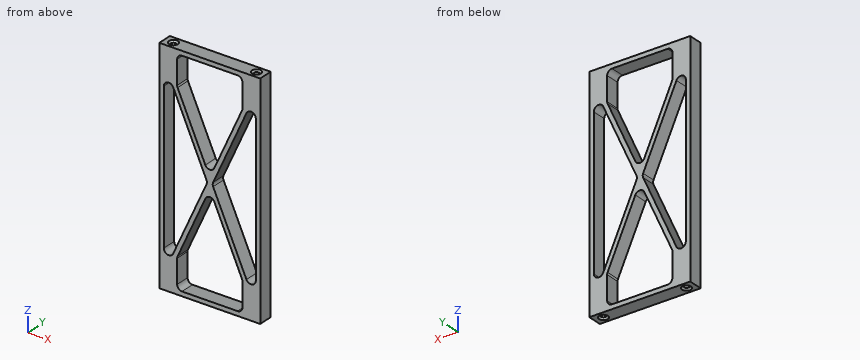
```python
from build123d import *

# Parameters (mm, degrees)
SKETCH1_W                       = 68
SKETCH1_H                       = 152.18109071
BOSS_EXTRUDE1_DEPTH             = 4.7625
CUT_EXTRUDE2_DEPTH              = 10.525
MIRROR3_COPY_1_DEPTH            = 10.525
FILLET1_R                       = 3.3
F_10_24_TAPPED_HOLE1_AT_2_COUNT = 2
F_10_24_TAPPED_HOLE1_AT_2_PITCH = 56


with BuildPart() as part:
    # Sketch1 → Boss-Extrude1 (new body, symmetric)
    with BuildSketch(Plane(origin=(0, 0, 0), x_dir=(1, 0, 0), z_dir=(0, 1, 0))):
        Rectangle(SKETCH1_W, SKETCH1_H)
    extrude(amount=BOSS_EXTRUDE1_DEPTH, both=True)

    # Sketch5 → Cut-Extrude2 (cut, through all)
    with BuildSketch(Plane(origin=(0, 4.7625, 0), x_dir=(1, 0, 0), z_dir=(0, 1, 0))):
        Polygon((-31, -65.699851963), (-31, 0), (-1.642936566, 0), align=None)
        Polygon((-22, -73.090545355), (0, -73.090545355), (0, -3.676821743), (-22, -52.911880502), align=None)
    cut_extrude2 = extrude(amount=-CUT_EXTRUDE2_DEPTH, mode=Mode.SUBTRACT)

    # Mirror2: Cut-Extrude2 across plane
    add(cut_extrude2.mirror(Plane(origin=(0, 0, 0), x_dir=(0, 0, 1), z_dir=(1, 0, 0))), mode=Mode.SUBTRACT)

    # Mirror3: Cut-Extrude2 across plane
    add(cut_extrude2.mirror(Plane.XY), mode=Mode.SUBTRACT)

    # Mirror3 copy 1 sketch → Mirror3 copy 1 (cut, through all)
    with BuildSketch(Plane(origin=(0, 4.7625, 0), x_dir=(-1, 0, 0), z_dir=(0, 1, 0))):
        Polygon((-31, -65.699851963), (-31, 0), (-1.642936566, 0), align=None)
        Polygon((-22, -73.090545355), (0, -73.090545355), (0, -3.676821743), (-22, -52.911880502), align=None)
    extrude(amount=-MIRROR3_COPY_1_DEPTH, mode=Mode.SUBTRACT)

    # Fillet1
    fillet1_edges = [part.edges().sort_by_distance(p)[0] for p in [
        (-1.642936566, 0, 0),
        (-31, 0, 65.699851963),
        (0, 0, 3.676821743),
        (-22, 0, 73.090545355),
        (-22, 0, 52.911880502),
        (31, 0, 65.699851963),
        (1.642936566, 0, 0),
        (22, 0, 52.911880502),
        (22, 0, 73.090545355),
        (31, 0, -65.699851963),
        (0, 0, -3.676821743),
        (22, 0, -73.090545355),
        (22, 0, -52.911880502),
        (-31, 0, -65.699851963),
        (-22, 0, -52.911880502),
        (-22, 0, -73.090545355),
    ]]
    fillet(fillet1_edges, radius=FILLET1_R)

    # Sketch2 → #10-24 Tapped Hole1 (revolve, cut)
    with BuildSketch(Plane(origin=(-28, 0, 76.090545355), x_dir=(0, -1, 0), z_dir=(1, 0, 0))):
        Polygon((0, 0), (0, 16.090824014), (1.89865, 14.95), (1.89865, 1.14935), (3.048, 0), align=None)
    f_10_24_tapped_hole1 = revolve(axis=Axis((-28, 0, 82.440545355), (0, 0, -1)), mode=Mode.SUBTRACT)

    # #10-24 Tapped Hole1 at 2: #10-24 Tapped Hole1 ×2
    with Locations(*[(i * F_10_24_TAPPED_HOLE1_AT_2_PITCH, 0, 0) for i in range(1, F_10_24_TAPPED_HOLE1_AT_2_COUNT)]):
        add(f_10_24_tapped_hole1, mode=Mode.SUBTRACT)

    # Mirror1: #10-24 Tapped Hole1 across plane
    add(f_10_24_tapped_hole1.mirror(Plane.XY), mode=Mode.SUBTRACT)

    # Mirror1 copy 1 sketch → Mirror1 copy 1 (revolve, cut)
    with BuildSketch(Plane(origin=(28, 0, -76.090545355), x_dir=(0, -1, 0), z_dir=(1, 0, 0))):
        Polygon((0, 0), (0, -16.090824014), (1.89865, -14.95), (1.89865, -1.14935), (3.048, 0), align=None)
    revolve(axis=Axis((28, 0, -82.440545355), (0, 0, -1)), mode=Mode.SUBTRACT)


solid = part.part
```
Read the model definition and answer for the solid it produces. Units are mm, in the model's axes. Coordinates: 2 decimals unless noted, no trailing zeros. Order: outer loops, then holes, each group sorted by start corner. A loop starts at its lowest first (then second) coordinate and runs counter-clockwise, first axis right, second up. Notation, with made-up numbers: (-9, 59.5) - (38, 59.5) arc R33 ccw to (38, 87.5) - close; hole circle Ø7 at (38, -8). An arc over 180 degrees is marked (long way). Answer as a JSON object with one key per item and string values. Group by question number.
Item 1: Section B-B (x = 13.5) is taken. Give the vertices of the cut face in (y, z).
Item 2: Section A-A (z = 56) is taken. Give the vertices of the cut face in (x, y).
Item 3: Consider probe 1 along Z at (x, y) = (0, 0.5); probe 2 along X at (y, z) = (0, -65); probe 3 along Z at (x, y) = (-3, -1.5). Determine where each line is inside the solid, lowest interval first. Write a range as from..to.
Item 4: Flat-ended cylindrical pins translate along their axes: P1, Ø4.5, axis at x = 28, y = 0, coming from the +Z side; P2, Ø5, axis at x = 28, y = 0, coming from the -Z side; P3, Ø5, axis at x = -28, y = 0, coming from the +Z side. Find the tip coordinate at first contact, or state that the pin passes through.
Results are:
{
 "1": {"outline": "(-4.76, -76.09) - (4.76, -76.09) - (4.76, -73.09) - (-4.76, -73.09) - close; (-4.76, -33.89) - (4.76, -33.89) - (4.76, -26.54) - (-4.76, -26.54) - close; (-4.76, 26.54) - (4.76, 26.54) - (4.76, 33.89) - (-4.76, 33.89) - close; (-4.76, 73.09) - (4.76, 73.09) - (4.76, 76.09) - (-4.76, 76.09) - close"},
 "2": {"outline": "(-34, -4.76) - (-22, -4.76) - (-22, 4.76) - (-34, 4.76) - close; (22, -4.76) - (34, -4.76) - (34, 4.76) - (22, 4.76) - close"},
 "3": {"probe 1": "z = -76.09..-73.09, -8.47..8.47, 73.09..76.09", "probe 2": "x = -34..-29.9, -26.1..-22, 22..26.1, 29.9..34", "probe 3": "z = -76.09..-73.09, -10.39..-3.04, 3.04..10.39, 73.09..76.09"},
 "4": {"P1": "stops at z = 75.29", "P2": "stops at z = -75.54", "P3": "stops at z = 75.54"}
}
